The model under review builds one solid part; all positions refer to its coordinate system, in mm. A direction names the side the tool comes from. Give positions to 0.01 mm unless a question says otherwise; leave off trailing zeros. Order: outer loops, then holes, each group sorted by start corner. A loop starts at its lowest first (then second) coordinate and runs counter-clockwise, first axis right, second up. Notation, with made-up numbers: (36.25, -13) - (76.25, -13) arc R30 cw to (76.25, 21) - close; hole circle Ø7 at (47, 64.5). An arc over 180 degrees is marked (long way). Use CSV: the item, a comma, the result in double quotes. Start each with the question number.
1. Take a section at D-D, the plane z = -7. State the section outline as (x, y) points.
2. Machinability: for faces 1 (the flat face through (-24, 10, 0)), 2 (the cylindrical face through (15.62, 16.53, 6.66)), 3 (the cylindrical face through (-16.707, 17.806, 4.666)), 4 (the flat face through (2.4, 3.8, 8)), 5 (the cylindrical face through (-29.747, 5.07, -0.121)), which of the approach directions +Z, -Z, +X, -X, +Y, -Y give a long, thin tool a straight path to every point of the face, cutting with its end or side? Answer none if there is none.
3. To check wall thickness, follow line 1 (X direction, y = 3.25, z = 0); line 2 (Y direction, x = 0, z = 3); line 3 (Y direction, x = 0, z = 4.9). State the ranges of each line that lie inside material, in increasing order. Write a range as [from, to].
4. For pin 1 (6.5 mm diameter, centred on x = -27, z = 0, fed in from -Y); pin 2 (4 mm diameter, centred on y = 16, z = 2, fed in from -X); pin 3 (1 mm diameter, centred on y = 17.5, z = -6, fed in from +X); pin 4 (3.5 mm diameter, centred on x = -28, z = 0.5, fed in from +Y), all flat-tipped, find the tip position at first contact; note any pin that passes through.
5. Draft analysis for pull direction Z (two halves, no side actions). For faces 6 (the cylindrical face through (15.437, 35.189, 0.112)), 7 (the flat face through (-8, 7, -8)), 8 (the flat face through (6, 35, 4)), state which applies: released by +Z, released by -Z, zero draft, split by the parting line, or undercut.
6. Take a section at B-B, the plane z = 0. State the section outline as (x, y) points, then the cut area to 3 significant figures.
7. Take a section at C-C, the plane x = -27. State the section outline as (y, z) points.
8. Take a section at A-A, the plane y = 20. State the section outline as (x, z) points, then the cut area to 3 significant figures.
```python
from build123d import *

# Parameters (mm, degrees)
EXTRUDE_1_DEPTH      = 8
EXTRUDE_1_DEPTH_BACK = 8
SKETCH_3_W           = 2.75
SKETCH_3_H           = 10
SKETCH_4_W           = 2.75
SKETCH_4_H           = 10


with BuildPart() as part:
    # Sketch 1 → Extrude 1 (new body, two sides)
    with BuildSketch(Plane.XY) as extrude_1_sk:
        with BuildLine():
            Line((-34, 9), (-34, 0))
            Line((-34, 0), (34, 0))
            Line((34, 0), (34, 9))
            ThreePointArc((34, 9), (33.707106781, 9.707106781), (33, 10))
            Line((33, 10), (21, 10))
            ThreePointArc((21, 10), (20.292893219, 10.292893219), (20, 11))
            Line((20, 11), (20, 24))
            ThreePointArc((20, 24), (15.313708499, 35.313708499), (4, 40))
            Line((4, 40), (-4, 40))
            ThreePointArc((-4, 40), (-15.313708499, 35.313708499), (-20, 24))
            Line((-20, 24), (-20, 11))
            ThreePointArc((-20, 11), (-20.292893219, 10.292893219), (-21, 10))
            Line((-21, 10), (-33, 10))
            ThreePointArc((-33, 10), (-33.707106781, 9.707106781), (-34, 9))
        make_face()
    extrude(amount=EXTRUDE_1_DEPTH)
    extrude(extrude_1_sk.sketch, amount=-EXTRUDE_1_DEPTH_BACK)

    # Sketch 2 → Cut-Revolve 1 (revolve, cut)
    with BuildSketch(Plane(origin=(0, 0, 0), x_dir=(0, 0, -1), z_dir=(1, 0, 0))):
        Polygon((-8, 20), (-8, 36), (-5.35, 36), (-5.35, 36.85), (-4, 36.85), (-4, 36), (6, 36), (6, 33), (8, 33), (8, 20), align=None)
    revolve(axis=Axis((0, 20, -8), (0, 0, 1)), mode=Mode.SUBTRACT)

    # Sketch 3 → Cut-Revolve 2 (revolve, cut)
    with BuildSketch(Plane.XY):
        with Locations((28.375, 5)):
            Rectangle(SKETCH_3_W, SKETCH_3_H)
    revolve(axis=Axis((27, 0, 0), (0, 1, 0)), mode=Mode.SUBTRACT)

    # Sketch 4 → Cut-Revolve 3 (revolve, cut)
    with BuildSketch(Plane.XY):
        with Locations((-25.625, 5)):
            Rectangle(SKETCH_4_W, SKETCH_4_H)
    revolve(axis=Axis((-27, 0, 0), (0, 1, 0)), mode=Mode.SUBTRACT)


solid = part.part
```
Determined:
1,outline,"(-34, 0) - (34, 0) - (34, 9) arc R1 ccw to (33, 10) - (21, 10) arc R1 cw to (20, 11) - (20, 24) arc R16 ccw to (4, 40) - (-4, 40) arc R16 ccw to (-20, 24) - (-20, 11) arc R1 cw to (-21, 10) - (-33, 10) arc R1 ccw to (-34, 9) - close; hole circle Ø26 at (0, 20)"
2,face 1,"+Z, -Z, -X, +Y"
2,face 2,"+Z"
2,face 3,"none"
2,face 4,"+Z, +X, -X, +Y, -Y"
2,face 5,"+Y, -Y"
3,line 1,"x = [-34, -29.75], [-24.25, 24.25], [29.75, 34]"
3,line 2,"y = [0, 4], [36, 40]"
3,line 3,"y = [0, 3.15], [36.85, 40]"
4,pin 1,"stops at y = 0"
4,pin 2,"stops at x = -20"
4,pin 3,"stops at x = 20"
4,pin 4,"stops at y = 10"
5,face 6,"zero draft"
5,face 7,"released by -Z"
5,face 8,"undercut"
6,outline,"(-34, 0) - (-29.75, 0) - (-29.75, 10) - (-33, 10) arc R1 ccw to (-34, 9) - close; (-24.25, 0) - (24.25, 0) - (24.25, 10) - (21, 10) arc R1 cw to (20, 11) - (20, 24) arc R16 ccw to (4, 40) - (-4, 40) arc R16 ccw to (-20, 24) - (-20, 11) arc R1 cw to (-21, 10) - (-24.25, 10) - close; (29.75, 0) - (34, 0) - (34, 9) arc R1 ccw to (33, 10) - (29.75, 10) - close; hole circle Ø32 at (0, 20)"
6,area,"856 mm²"
7,outline,"(0, -8) - (10, -8) - (10, -2.75) - (0, -2.75) - close; (0, 2.75) - (10, 2.75) - (10, 8) - (0, 8) - close"
8,outline,"(-20, -8) - (-13, -8) - (-13, -6) - (-16, -6) - (-16, 4) - (-16.85, 4) - (-16.85, 5.35) - (-16, 5.35) - (-16, 8) - (-20, 8) - close; (13, -8) - (20, -8) - (20, 8) - (16, 8) - (16, 5.35) - (16.85, 5.35) - (16.85, 4) - (16, 4) - (16, -6) - (13, -6) - close"
8,area,"138 mm²"
